Geometry: see drawing. Coordinates: mm, zero at the bounding-box minimum. A direction names the side the tool comes from. Coordinates: 2 decimals unless noted, no trailing zeros. Loops run counter-clockwise (first coordinate to the right, second up) from the corner with the lowest first, then second, coordinate; pieces in that order, holes last. Notation, with made-up numbers: (88, 64) -> (108, 64) arc R10 ccw to (108, 82) -> close; hole circle Ø5 at (1, 1.5). An arc over 180 degrees is marked (long way). One line per question, with ' | ' between items. Start each with the question number.
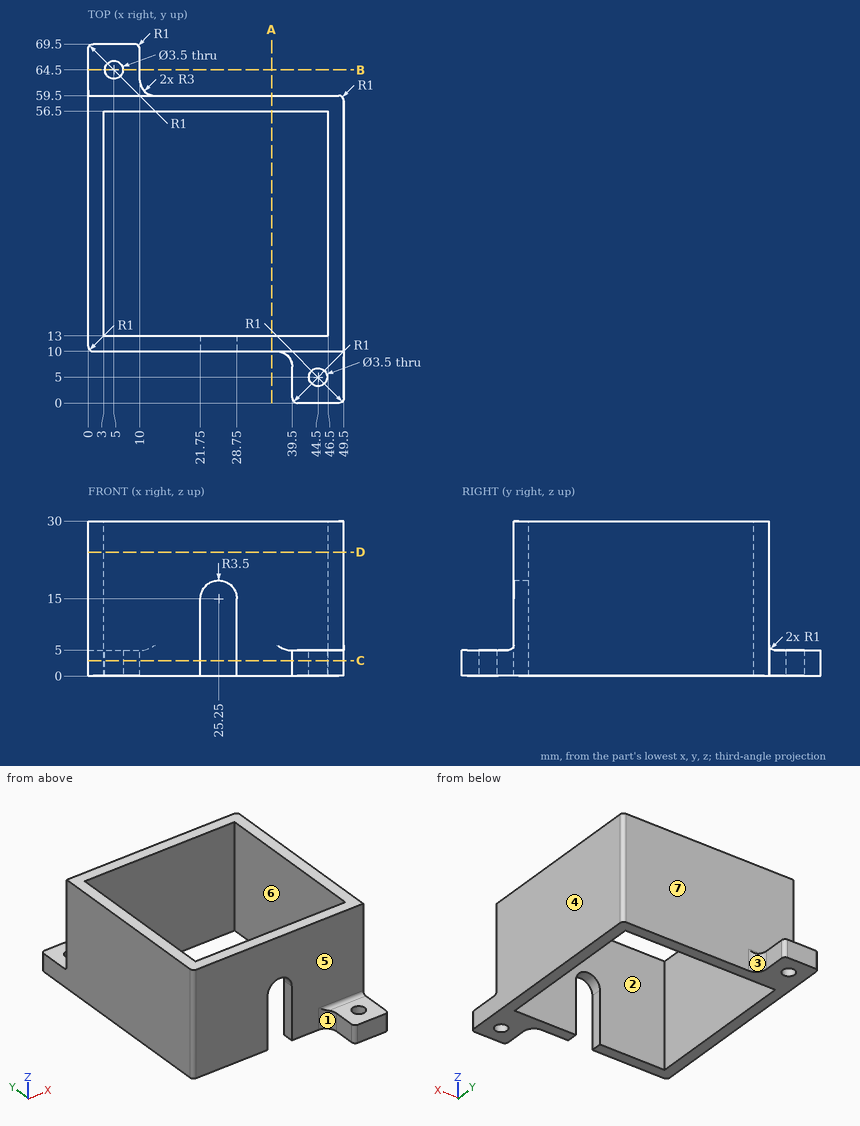
(1) Cut plane C-C, the plane z = 3. Return the cut outline in (x, y), and give its area (3 significant figures).
(2) Draft query along Y for the marked faces 1, 2 and 3. Return one class per face: pulls with the +Y half, pulls with the -Y half, needs draft (parallel to the pull), parting line crosses it, or undercut.
(3) Cut plane A-A, the plane x = 35.5. Return the cut outline in (y, z).
(4) Contact query for flat-ended pins moving along their axis: pin 1 Ø6 at (x, y) = (43, 27.5) entering from -Z; pin 2 Ø10 at (x, y) = (43.5, 3) entering from +Z; pin 3 Ø5.5 at (y, z) = (4.5, 3.5) entering from -X; pin 4 Ø3 at (x, z) = (10.5, 16) entering from +Y. Output: stop coordinate, or through.
(5) Access query for the marked faces 4, 5, 6 and 7. Directions: +Z, -Z, +X, -X, +Y, -Y. A direction counts if a zero-diameter tool reaches every point of the face in a straight line with its end or side. Return the directions, or none.
(6) Ray query, L1, parallel to Y at x = 5, z = 1.6; L2, parallel to Y at x = 44.5, z = 3.05; L3, parallel to X at y = 41, z = 9.5. Return the intervals inside material, ascending.
(7) Cut plane D-D, the plane z = 24. Return the cut outline in (x, y), and give its area (3 significant figures).
(8) Cut plane B-B, the plane y = 64.5. Return the cut outline in (x, z).
Here are the results:
1) outline: (0, 11) arc R1 ccw to (1, 10) -> (21.75, 10) -> (21.75, 13) -> (3, 13) -> (3, 56.5) -> (46.5, 56.5) -> (46.5, 13) -> (28.75, 13) -> (28.75, 10) -> (36.5, 10) arc R3 cw to (39.5, 7) -> (39.5, 1) arc R1 ccw to (40.5, 0) -> (48.5, 0) arc R1 ccw to (49.5, 1) -> (49.5, 58.5) arc R1 ccw to (48.5, 59.5) -> (13, 59.5) arc R3 cw to (10, 62.5) -> (10, 68.5) arc R1 ccw to (9, 69.5) -> (1, 69.5) arc R1 ccw to (0, 68.5) -> close; hole circle Ø3.5 at (5, 64.5); hole circle Ø3.5 at (44.5, 5) | area: 720 mm2
2) face 1: pulls with the -Y half | face 2: undercut | face 3: pulls with the +Y half
3) outline: (10, 0) -> (13, 0) -> (13, 30) -> (10, 30) -> close; (56.5, 0) -> (59.5, 0) -> (59.5, 30) -> (56.5, 30) -> close
4) pin 1: passes through | pin 2: stops at z = 5 | pin 3: stops at x = 39.49 | pin 4: stops at y = 59.5
5) face 4: +Z, -Z, +X, +Y, -Y | face 5: +Z, -X, -Y | face 6: +Z, -Z | face 7: +Z, +X, +Y
6) L1: y = 10 to 13, 56.5 to 62.75, 66.25 to 69.5 | L2: y = 0 to 3.25, 6.75 to 13, 56.5 to 59.5 | L3: x = 0 to 3, 46.5 to 49.5
7) outline: (0, 11) arc R1 ccw to (1, 10) -> (49.5, 10) -> (49.5, 58.5) arc R1 ccw to (48.5, 59.5) -> (0, 59.5) -> close; hole (3, 13) -> (46.5, 13) -> (46.5, 56.5) -> (3, 56.5) -> close | area: 558 mm2
8) outline: (0, 0) -> (3.25, 0) -> (3.25, 5) -> (0, 5) -> close; (6.75, 0) -> (10, 0) -> (10, 5) -> (6.75, 5) -> close
